from build123d import *

# Parameters (mm, degrees)
F1_DEPTH = 5
F2_DEPTH = 30
F3_DEPTH = 30
F4_DEPTH = 30
F5_R     = 10
F6_DEPTH = 40


with BuildPart() as f1:
    # F0 (on Top) → F1 (new body)
    with BuildSketch(Plane.XY):
        with BuildLine():
            Line((32.5, 0), (32.5, 7.5))
            Line((32.5, 7.5), (25, 7.5))
            ThreePointArc((25, 7.5), (30.303301, 5.303301), (32.5, 0))
        make_face()
        with BuildLine():
            ThreePointArc((25, -7.5), (17.5, 0), (25, 7.5))
            Line((25, 7.5), (0, 7.5))
            ThreePointArc((0, 7.5), (5.303301, 5.303301), (7.5, 0))
            ThreePointArc((7.5, 0), (5.303301, -5.303301), (0, -7.5))
            Line((0, -7.5), (25, -7.5))
        make_face()
        with BuildLine():
            Line((32.5, -7.5), (32.5, 0))
            ThreePointArc((32.5, 0), (30.303301, -5.303301), (25, -7.5))
            Line((25, -7.5), (32.5, -7.5))
        make_face()
        with BuildLine():
            ThreePointArc((-7.5, 0), (-5.303301, 5.303301), (0, 7.5))
            Line((0, 7.5), (-25, 7.5))
            ThreePointArc((-25, 7.5), (-19.696699, 5.303301), (-17.5, 0))
            Line((-17.5, 0), (-7.5, 0))
        make_face()
        with BuildLine():
            ThreePointArc((-32.5, 0), (-30.303301, 5.303301), (-25, 7.5))
            Line((-25, 7.5), (-32.5, 7.5))
            Line((-32.5, 7.5), (-32.5, 0))
        make_face()
        with BuildLine():
            ThreePointArc((0, -7.5), (-5.303301, -5.303301), (-7.5, 0))
            Line((-7.5, 0), (-17.5, 0))
            ThreePointArc((-17.5, 0), (-19.696699, -5.303301), (-25, -7.5))
            Line((-25, -7.5), (0, -7.5))
        make_face()
        with BuildLine():
            ThreePointArc((-25, -7.5), (-30.303301, -5.303301), (-32.5, 0))
            Line((-32.5, 0), (-32.5, -7.5))
            Line((-32.5, -7.5), (-25, -7.5))
        make_face()
    extrude(amount=F1_DEPTH)

    # F0 (on Top) → F2 (join)
    with BuildSketch(Plane.XY):
        with BuildLine():
            ThreePointArc((-17.5, 0), (-19.696699, 5.303301), (-25, 7.5))
            ThreePointArc((-25, 7.5), (-30.303301, 5.303301), (-32.5, 0))
            ThreePointArc((-32.5, 0), (-30.303301, -5.303301), (-25, -7.5))
            ThreePointArc((-25, -7.5), (-19.696699, -5.303301), (-17.5, 0))
        make_face()
    extrude(amount=F2_DEPTH)

    # F0 (on Top) → F3 (join)
    with BuildSketch(Plane.XY):
        with BuildLine():
            ThreePointArc((7.5, 0), (5.303301, 5.303301), (0, 7.5))
            ThreePointArc((0, 7.5), (-5.303301, 5.303301), (-7.5, 0))
            ThreePointArc((-7.5, 0), (-5.303301, -5.303301), (0, -7.5))
            ThreePointArc((0, -7.5), (5.303301, -5.303301), (7.5, 0))
        make_face()
    extrude(amount=F3_DEPTH)

    # F0 (on Top) → F4 (join)
    with BuildSketch(Plane.XY):
        with BuildLine():
            ThreePointArc((32.5, 0), (30.303301, 5.303301), (25, 7.5))
            ThreePointArc((25, 7.5), (17.5, 0), (25, -7.5))
            ThreePointArc((25, -7.5), (30.303301, -5.303301), (32.5, 0))
        make_face()
    extrude(amount=F4_DEPTH)

    # F5 (on face) → F6 (join)
    with BuildSketch(Plane(origin=(0, 0, 0), x_dir=(1, 0, 0), z_dir=(0, 0, -1))):
        Circle(F5_R)
    extrude(amount=F6_DEPTH)


solid = f1.part
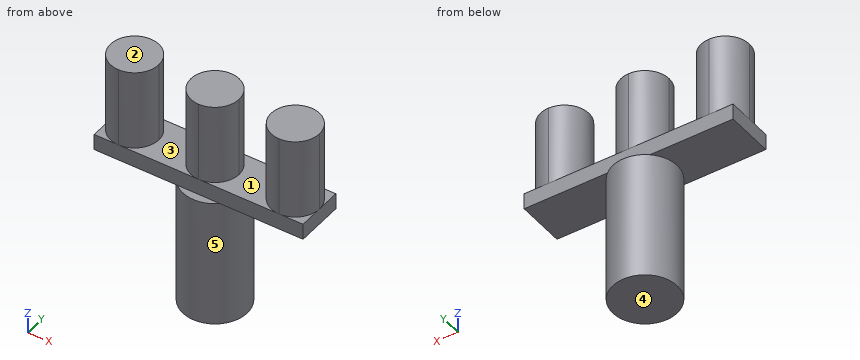
The listing builds one solid part. Answer for the finished solid, in the listing's coordinates (mm). Face numbers are marked on the shaded views. A direction names the side the tool comes from. Give positions to 0.01 mm unless a question says otherwise; leave off trailing zeros. Write each loop counter-clockwise with the first axis right and the second up, starting at its lowest first coordinate (ties: lowest second). Pieces come first, ordered by that corner, then holes. Notation, with made-up numbers: (73.25, 27) -> (127.25, 27) arc R26 ccw to (127.25, 52) -> close; hole circle Ø5 at (73, -17.75). An arc over 180 degrees is marked (long way). One line per question, with ' | ' between items. Start each with the question number.
1. Section B-B (y = 6) is taken. Determine the outline of the cut face in (x, z).
2. For the marked faces 1 and 2, determine the directions among +Z, -Z, +X, -X, +Y, -Y from which every point of the face is accessible in a straight line to the end or side of a thin tool.
3. Given pin 1 Ø6 at (x, z) = (-17.5, 17) entering from +Y; pin 2 Ø2.5 at (x, z) = (-4, 2) entering from +Y; pin 3 Ø2.5 at (x, z) = (13.5, 3.5) entering from -Y; pin 4 Ø4 at (x, z) = (10, 14.5) entering from -Y, each flat-ended and moving along its own axis, determine where each tip first touches the part or whether it passes through.
4. Find the intervals of material crossed by probe 1 along X at (y, z) = (4.5, 19); probe 2 along X at (y, z) = (6.75, 8); probe 3 along Z at (x, y) = (-1.5, 8.75), in increasing order.
5. Section A-A (z = 12) is taken. Determine the outline of the cut face in (x, y), plus the area to 3 significant figures.
6. Section D-D (z = -35) is taken. Determine the outline of the cut face in (x, y), plus the area to 3 significant figures.
7. Section C-C (x = -22.5) is taken. Determine the outline of the cut face in (y, z).
8. For a pull along X with two mould halves and no side action, classify the marked faces 3, 4 and 5 as pulls with the +X half, pulls with the -X half, needs draft (parallel to the pull), parting line crosses it, or undercut.
Response values:
1) outline: (-32.5, 0) -> (-8, 0) -> (-8, -40) -> (8, -40) -> (8, 0) -> (32.5, 0) -> (32.5, 5) -> (29.5, 5) -> (29.5, 30) -> (20.5, 30) -> (20.5, 5) -> (4.5, 5) -> (4.5, 30) -> (-4.5, 30) -> (-4.5, 5) -> (-20.5, 5) -> (-20.5, 30) -> (-29.5, 30) -> (-29.5, 5) -> (-32.5, 5) -> close
2) face 1: +Z | face 2: +Z, +X, -X, +Y, -Y
3) pin 1: y = 6 | pin 2: y = 7.5 | pin 3: y = -7.5 | pin 4: through
4) probe 1: -31 to -19, -6 to 6, 19 to 31 | probe 2: -28.27 to -21.73, -3.27 to 3.27, 21.73 to 28.27 | probe 3: -40 to 0
5) outline: circle Ø15 at (-25, 0); circle Ø15 at (0, 0); circle Ø15 at (25, 0) | area: 530 mm2
6) outline: circle Ø20 at (0, 0) | area: 314 mm2
7) outline: (-7.5, 0) -> (7.5, 0) -> (7.5, 5) -> (7.07, 5) -> (7.07, 30) -> (-7.07, 30) -> (-7.07, 5) -> (-7.5, 5) -> close
8) face 3: undercut | face 4: needs draft | face 5: parting line crosses it
